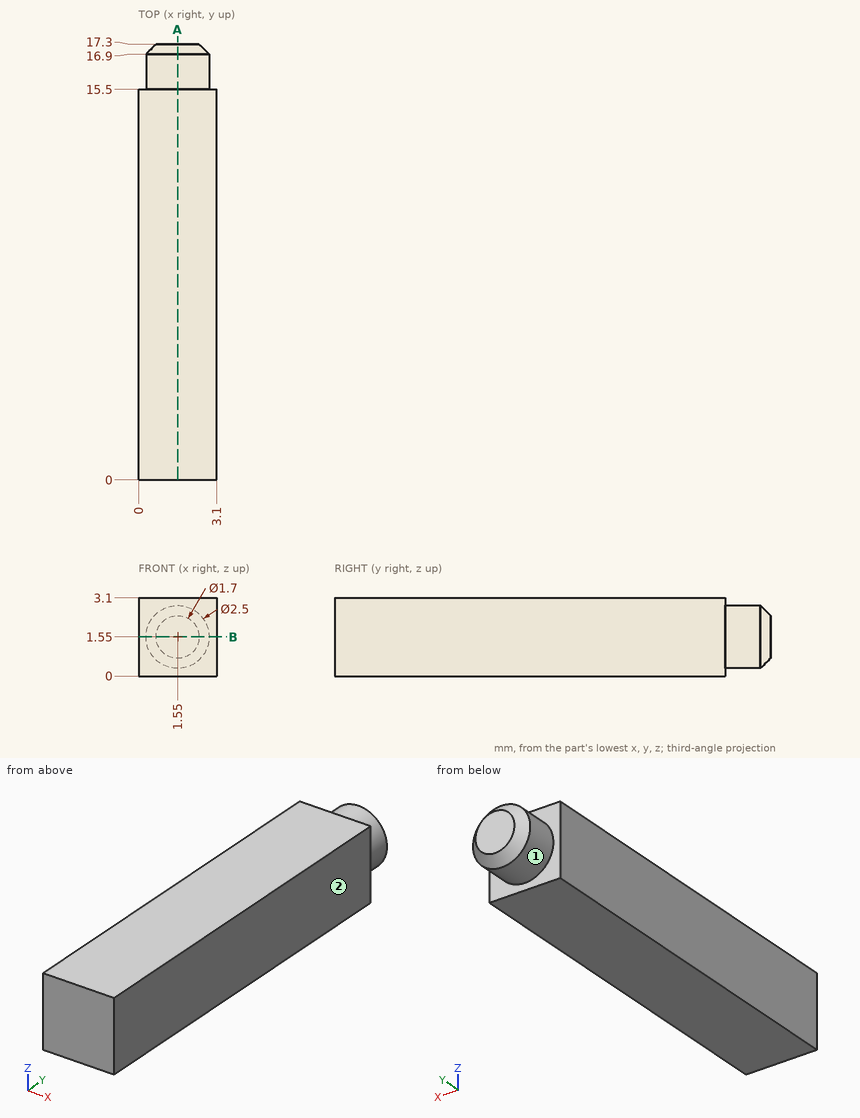
Geometry: see drawing. Coordinates: mm, zero at the bounding-box minimum. A direction names the side the tool comes from. Coordinates: 2 decimals unless noted, no trailing zeros. Order: outer loops, then holes, each group sorted by start corner. A loop starts at its lowest first (then second) coordinate and runs counter-clockwise, first axis right, second up. Notation, with made-up numbers: (34, 43) -> (76, 43) arc R21 cw to (76, 56) -> close; hole circle Ø7 at (3.5, -36.75). An arc over 180 degrees is marked (long way). Write each question's results on one line, items separated by ' | '. Start each with the question number.
1) Set-up query: the marked faces 1 and 2. Return all of +Z, -Z, +X, -X, +Y, -Y with unobstructed straight access to the full face (end or side cutting, diameter ignored); none if empty.
2) Cut plane B-B, the plane z = 1.55. Output: boundary loops of the cut face in (x, y), and give its area (3 significant figures).
3) Material intervals for line 1 along Y through (x, z) = (0.45, 0.45); line 2 along Y through (x, z) = (2, 0.45); line 3 along Z through (x, y) = (2.4, 15.75), sorted ascending.
4) Cut plane A-A, the plane x = 1.55. Output: boundary loops of the cut face in (y, z).
Checks:
1) face 1: +Y | face 2: +Z, -Z, +X, +Y, -Y
2) outline: (0, 0) -> (3.1, 0) -> (3.1, 15.5) -> (2.8, 15.5) -> (2.8, 16.9) -> (2.4, 17.3) -> (0.7, 17.3) -> (0.3, 16.9) -> (0.3, 15.5) -> (0, 15.5) -> close | area: 52.4 mm^2
3) line 1: 0 to 15.5 | line 2: 0 to 16.96 | line 3: 0.63 to 2.47
4) outline: (0, 0) -> (15.5, 0) -> (15.5, 0.3) -> (16.9, 0.3) -> (17.3, 0.7) -> (17.3, 2.4) -> (16.9, 2.8) -> (15.5, 2.8) -> (15.5, 3.1) -> (0, 3.1) -> close
